Drawing for the job (mm, zero at the part's lowest x, y, z). A direction names the side the tool comes from. Coordinates: 2 decimals unless noted, no trailing zeros. Order: outer loops, then holes, each group sorted by start corner. A loop starts at its lowest first (then second) coordinate and runs counter-clockwise, first axis right, second up.
1) Pin check, flat tips, straight feed: pin 1 Ø1 at (x, z) = (9.5, 9.5) entering from -Y; pin 2 Ø5 at (x, z) = (16.5, 17.5) entering from -Y (3 decimals); pin 3 Ø5 at (y, z) = (14, 15.5) entering from +X (3 decimals); pin 4 Ø3 at (x, z) = (12, 22.5) entering from +Y. Stop position of each tip, or through.
2) Cut at D-D (x = 5.5). List the corners of the cut face in (y, z) (3 decimals), and give its area (3 significant figures).
3) Tool access for the marked faces 1, 2 and 3: list every direction of +Z, -Z, +X, -X, +Y, -Y with a clear straight run to the whole face (end or side of a thin tool).
4) Cut at C-C (z = 22.75). List the corners of the cut face in (x, y).
5) Wall check: L1, parallel to Y at x = 12, z = 14 (3 decimals); L2, parallel to X at y = 19, z = 23. Give the ranges that are in metal, low to high.
6) Cut at A-A (x = 12.25). List the corners of the cut face in (y, z) (3 decimals).
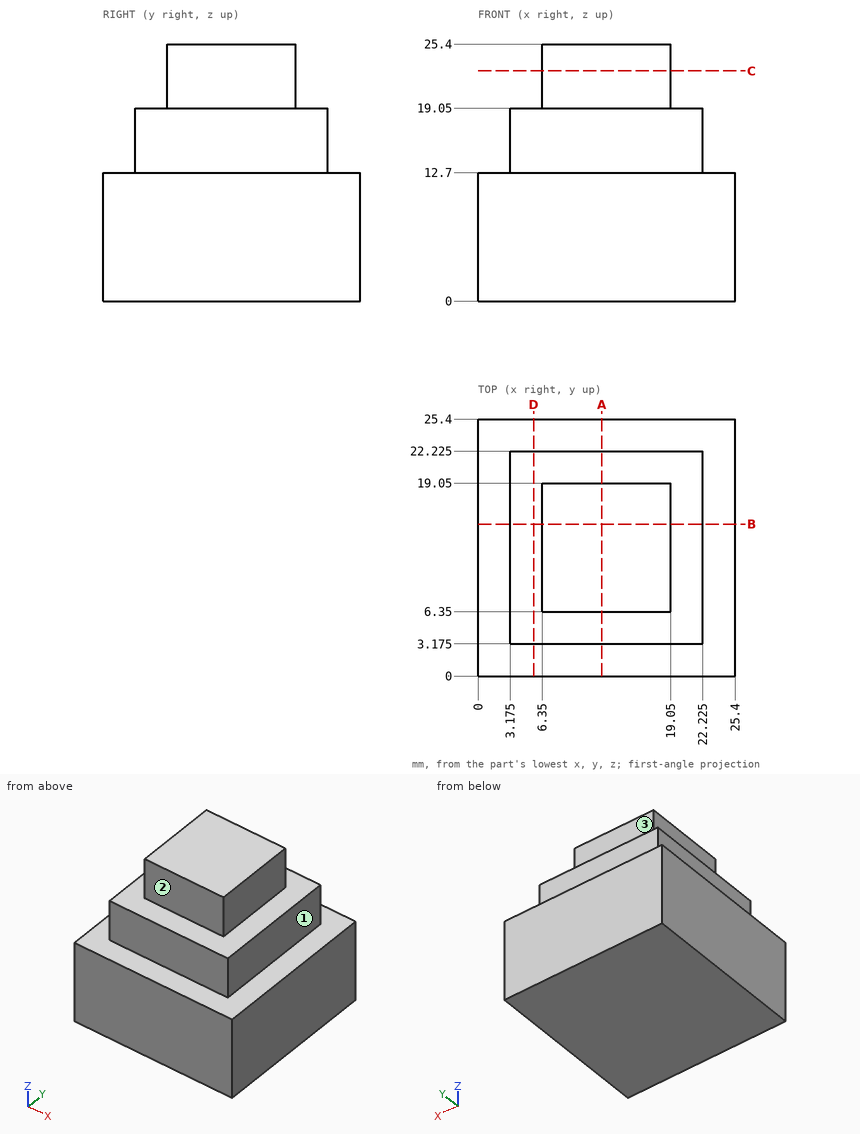
Geometry check:
1. pin 1: stops at y = 0
1. pin 2: stops at y = 3.175
1. pin 3: stops at x = 22.225
1. pin 4: stops at y = 19.05
2. outline: (0, 0) - (25.4, 0) - (25.4, 12.7) - (22.225, 12.7) - (22.225, 19.05) - (3.175, 19.05) - (3.175, 12.7) - (0, 12.7) - close
2. area: 444 mm2
3. face 1: +Z, +X, +Y, -Y
3. face 2: +Z, +X, -X, -Y
3. face 3: +Z, +X, -X, +Y
4. outline: (6.35, 6.35) - (19.05, 6.35) - (19.05, 19.05) - (6.35, 19.05) - close
5. L1: y = 3.175 to 22.225
5. L2: x = 6.35 to 19.05
6. outline: (0, 0) - (25.4, 0) - (25.4, 12.7) - (22.225, 12.7) - (22.225, 19.05) - (19.05, 19.05) - (19.05, 25.4) - (6.35, 25.4) - (6.35, 19.05) - (3.175, 19.05) - (3.175, 12.7) - (0, 12.7) - close
